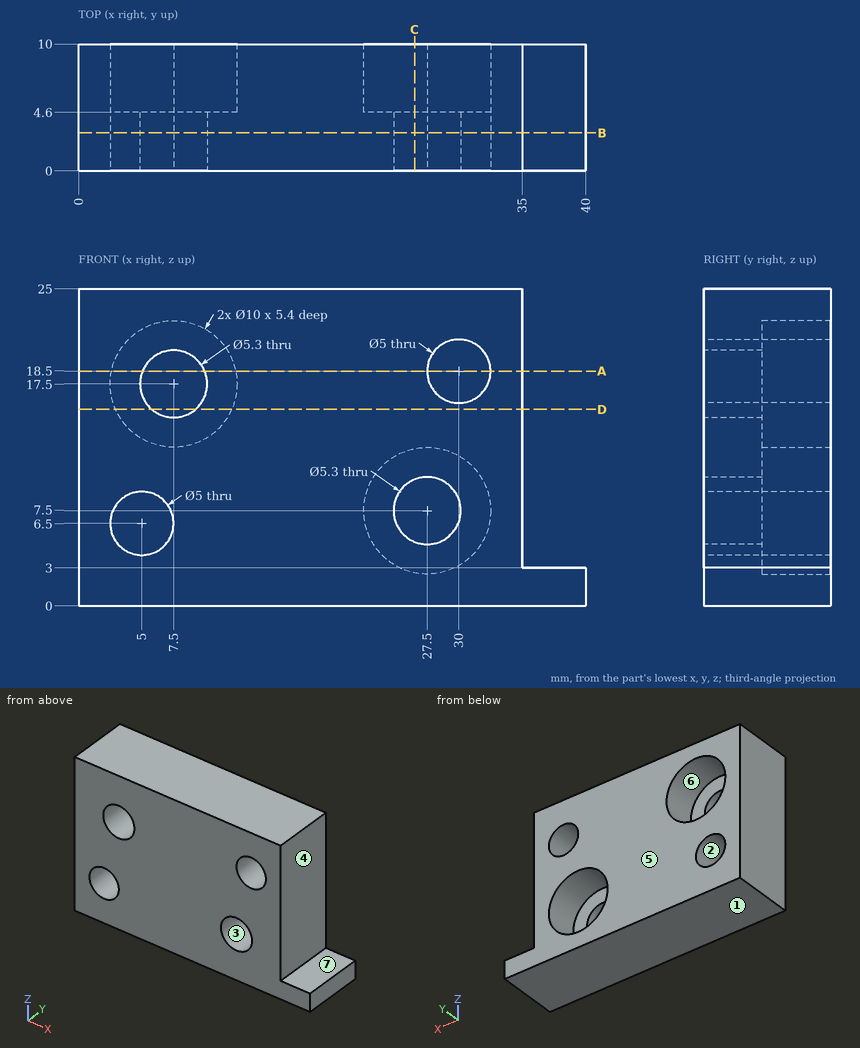
Job drawing, mm, ordinate dimensions from the low corner. One solid piece. A direction names the side the tool comes from. Coordinates: 2 decimals unless noted, no trailing zeros. Loops run counter-clockwise (first coordinate to the right, second up) from the corner with the lowest first, then second, coordinate; pieces in that order, holes last. Notation, with made-up numbers: (12.25, 55.5) - (65.25, 55.5) arc R27 cw to (65.25, 74.5) - close; hole circle Ø9 at (63.25, -29). An arc over 180 degrees is marked (long way). Write item = value, one per line. Start each with the question number.
Q1. Cut at B-B, the plane y = 3. List the corners of the cut face in (x, z), then the cut area to 3 significant figures.
Q2. Which spindle directions (+Z, -Z, +X, -X, +Y, -Y) get a long thin tool onto all of the face, cutting with end or side? Do the marked faces 5, 6 and 7. Say none if no direction does.
Q3. Cut at C-C, the plane x = 26.5. List the corners of the cut face in (y, z), then the cut area to 3 significant figures.
Q4. Pull direction Z, two halves, no side cores. Call the marked faces 1, 2, 3 and 4: pulls with the +Z half, pulls with the -Z half, needs draft (parallel to the pull), parting line crosses it, or undercut.
Q5. Cut at D-D, the plane z = 15.5. List the corners of the cut face in (x, y).
Q6. Cut at A-A, the plane z = 18.5. List the corners of the cut face in (x, y).
Q7. Flat gauge pins, fed straight in: pin 1 Ø1.5 at (x, y) = (37.5, 5.5) entering from +Z; pin 2 Ø8 at (x, z) = (7.5, 17.5) entering from +Y. Where does each tip first touch, or does it go through?
Q8. Drill centre lines: L1, parallel to X at y = 9.75, z = 4.25; L2, parallel to Z at x = 3, y = 6.75; L3, parallel to X at y = 4, z = 5.25. Where is each one in solid material? Low to high.
Computed:
q1.outline = (0, 0) - (40, 0) - (40, 3) - (35, 3) - (35, 25) - (0, 25) - close; hole circle Ø5 at (5, 6.5); hole circle Ø5.3 at (7.5, 17.5); hole circle Ø5.3 at (27.5, 7.5); hole circle Ø5 at (30, 18.5)
q1.area = 807 mm²
q2.face_5 = +Z, -Z, +X, -X, +Y
q2.face_6 = +Y
q2.face_7 = +Z, +X, +Y, -Y
q3.outline = (0, 0) - (10, 0) - (10, 2.6) - (4.6, 2.6) - (4.6, 5.05) - (0, 5.05) - close; (0, 9.95) - (4.6, 9.95) - (4.6, 12.4) - (10, 12.4) - (10, 25) - (0, 25) - close
q3.area = 175 mm²
q4.face_1 = pulls with the -Z half
q4.face_2 = undercut
q4.face_3 = undercut
q4.face_4 = needs draft
q5.outline = (0, 0) - (5.76, 0) - (5.76, 4.6) - (2.92, 4.6) - (2.92, 10) - (0, 10) - close; (9.24, 0) - (35, 0) - (35, 10) - (12.08, 10) - (12.08, 4.6) - (9.24, 4.6) - close
q6.outline = (0, 0) - (5.05, 0) - (5.05, 4.6) - (2.6, 4.6) - (2.6, 10) - (0, 10) - close; (9.95, 0) - (27.5, 0) - (27.5, 10) - (12.4, 10) - (12.4, 4.6) - (9.95, 4.6) - close; (32.5, 0) - (35, 0) - (35, 10) - (32.5, 10) - close
q7.pin_1 = 3
q7.pin_2 = 4.6
q8.L1 = 0 to 3.91, 6.09 to 23.7, 31.3 to 35
q8.L2 = 0 to 5, 8 to 15.32, 19.68 to 25
q8.L3 = 0 to 2.83, 7.17 to 26.1, 28.9 to 35
